from build123d import *

# Parameters (mm, degrees)
SKETCH1_R               = 3.25
BOSS_EXTRUDE1_DEPTH     = 1
SKETCH3_R               = 4.5
BOSS_EXTRUDE2_DEPTH     = 8
SKETCH4_W               = 43
SKETCH4_H               = 43
BOSS_EXTRUDE3_DEPTH     = 9
FILLET1_R               = 6
SKETCH5_R               = 12
BOSS_EXTRUDE4_DEPTH     = 14
CUT_EXTRUDE1_START      = 7
SKETCH6_R               = 12
SKETCH6_R_2             = 11
CUT_EXTRUDE1_DEPTH      = 1
BOSS_EXTRUDE5_DEPTH     = 3.5
FILLET2_R               = 4
SKETCH8_R               = 12
BOSS_EXTRUDE6_DEPTH     = 9
CHAMFER1_SIZE           = 1
BOSS_EXTRUDE7_START     = 10
SKETCH10_R              = 12
BOSS_EXTRUDE7_DEPTH     = 10
BOSS_EXTRUDE8_DEPTH     = 5
SKETCH12_R              = 12
BOSS_EXTRUDE9_DEPTH     = 48.5
CUT_EXTRUDE2_DEPTH      = 72.827221304
CUT_EXTRUDE2_DEPTH_BACK = 20
SKETCH13_W              = 26.789167307
SKETCH13_H              = 48.357994596
CHAMFER2_SIZE           = 1
CHAMFER4_SIZE           = 1
CHAMFER5_SIZE           = 1
SKETCH17_R              = 1.25
CUT_EXTRUDE4_DEPTH      = 88.387187875
CUT_EXTRUDE5_REACH      = 79.888
SKETCH18_R              = 3
SKETCH19_R              = 1.5
CUT_EXTRUDE6_DEPTH      = 53.140487552


with BuildPart() as part:
    # Sketch1 → Boss-Extrude1 (new body)
    with BuildSketch(Plane(origin=(0, 0, 0), x_dir=(1, 0, 0), z_dir=(0, 1, 0))):
        with BuildLine():
            Line((-17.5, -21.5), (17.5, -21.5))
            ThreePointArc((17.5, -21.5), (20.328427125, -20.328427125), (21.5, -17.5))
            Line((21.5, -17.5), (21.5, 17.5))
            ThreePointArc((21.5, 17.5), (20.328427125, 20.328427125), (17.5, 21.5))
            Line((17.5, 21.5), (-17.5, 21.5))
            ThreePointArc((-17.5, 21.5), (-20.328427125, 20.328427125), (-21.5, 17.5))
            Line((-21.5, 17.5), (-21.5, -17.5))
            ThreePointArc((-21.5, -17.5), (-20.328427125, -20.328427125), (-17.5, -21.5))
        make_face()
        with Locations(Location((-17.25, 17.25, 0), (0, 0, 270))):
            Circle(SKETCH1_R, mode=Mode.SUBTRACT)
        with Locations(Location((17.25, 17.25, 0), (0, 0, 270))):
            Circle(SKETCH1_R, mode=Mode.SUBTRACT)
        with Locations(Location((17.25, -17.25, 0), (0, 0, 270))):
            Circle(SKETCH1_R, mode=Mode.SUBTRACT)
        with Locations(Location((-17.25, -17.25, 0), (0, 0, 270))):
            Circle(SKETCH1_R, mode=Mode.SUBTRACT)
    extrude(amount=BOSS_EXTRUDE1_DEPTH)

    # Sketch3 → Boss-Extrude2 (add)
    with BuildSketch(Plane.XZ):
        with Locations(Location((-17.25, 17.25, 0), (0, 0, 70.811863546))):
            Circle(SKETCH3_R)
        with Locations(Location((17.25, 17.25, 0), (0, 0, 109.188136454))):
            Circle(SKETCH3_R)
        with Locations(Location((17.25, -17.25, 0), (0, 0, 19.188136454))):
            Circle(SKETCH3_R)
        with Locations(Location((-17.25, -17.25, 0), (0, 0, 160.811863546))):
            Circle(SKETCH3_R)
    extrude(amount=BOSS_EXTRUDE2_DEPTH)

    # Sketch4 → Boss-Extrude3 (add)
    with BuildSketch(Plane.XZ.offset(8)):
        Rectangle(SKETCH4_W, SKETCH4_H)
    extrude(amount=BOSS_EXTRUDE3_DEPTH)

    # Fillet1
    # the kernel refuses this fillet: 6 mm, written as the material it takes off along each edge
    with BuildSketch(Plane(origin=(-21.5, -8, 21.5), x_dir=(1, 0, 0), z_dir=(0, -1, 0)), Plane(origin=(-21.5, -8, -21.5), x_dir=(0, 0, 1), z_dir=(0, -1, 0)), Plane(origin=(21.5, -8, 21.5), x_dir=(0, 0, -1), z_dir=(0, -1, 0))) as fillet1_piece_1:
        with BuildLine():
            CenterArc((FILLET1_R, -FILLET1_R), FILLET1_R, 90, 90)
            Line((0, -FILLET1_R), (0, 0))
            Line((0, 0), (FILLET1_R, 0))
        make_face()
    extrude(amount=24, mode=Mode.SUBTRACT)
    with BuildSketch(Plane(origin=(21.5, -8, -21.5), x_dir=(0, 0, 1), z_dir=(0, -1, 0))) as fillet1_piece_2:
        with BuildLine():
            CenterArc((FILLET1_R, FILLET1_R), FILLET1_R, 180, 90)
            Line((0, FILLET1_R), (0, 0))
            Line((0, 0), (FILLET1_R, 0))
        make_face()
    extrude(amount=24, mode=Mode.SUBTRACT)

    # Sketch5 → Boss-Extrude4 (add)
    with BuildSketch(Plane.XZ.offset(17)):
        with Locations(Location((0, 0, 0), (0, 0, 270))):
            Circle(SKETCH5_R)
    extrude(amount=BOSS_EXTRUDE4_DEPTH)

    # Sketch6 → Cut-Extrude1 (cut)
    with BuildSketch(Plane.XZ.offset(17).offset(CUT_EXTRUDE1_START)):
        with Locations(Location((0, 0, 0), (0, 0, 270))):
            Circle(SKETCH6_R)
        with Locations(Location((0, 0, 0), (0, 0, 270))):
            Circle(SKETCH6_R_2, mode=Mode.SUBTRACT)
    extrude(amount=CUT_EXTRUDE1_DEPTH, mode=Mode.SUBTRACT)

    # Sketch7 → Boss-Extrude5 (add, symmetric)
    with BuildSketch(Plane(origin=(0, 0, 0), x_dir=(0, 0, -1), z_dir=(1, 0, 0))):
        Polygon((0, -25), (14.368756657, -25), (27.527515604, -41), (27.527515604, -66.788625846), (18.527515604, -66.788625846), (18.527515604, -41), (12, -31), (0, -31), align=None)
    extrude(amount=BOSS_EXTRUDE5_DEPTH, both=True)

    # Fillet2
    fillet2_edges = [part.edges().sort_by_distance(p)[0] for p in [
        (0, -31, -12),
    ]]
    fillet(fillet2_edges, radius=FILLET2_R)

    # Sketch8 → Boss-Extrude6 (add)
    with BuildSketch(Plane.XY.offset(-18.527515604)):
        with Locations((0, -55.310385562)):
            Circle(SKETCH8_R)
    extrude(amount=-BOSS_EXTRUDE6_DEPTH)

    # Chamfer1
    chamfer1_edges = [part.edges().sort_by_distance(p)[0] for p in [
        (0, -67.310385562, -18.527515604),
    ]]
    chamfer(chamfer1_edges, length=CHAMFER1_SIZE)

    # Sketch10 → Boss-Extrude7 (add)
    with BuildSketch(Plane.XY.offset(-18.527515604).offset(BOSS_EXTRUDE7_START)):
        with Locations(Location((0, -55.310385562, 0), (0, 0, 106.9577633))):
            Circle(SKETCH10_R)
    extrude(amount=-BOSS_EXTRUDE7_DEPTH)

    # Sketch11 → Boss-Extrude8 (add, symmetric)
    with BuildSketch(Plane(origin=(0, -55.310385562, 0), x_dir=(1, 0, 0), z_dir=(0, 1, 0))):
        Polygon((-13.638649199, -5.352201133), (-13.638649199, 8.527515604), (13.150518108, 8.527515604), (13.150518108, -5.352201133), (23.153950462, -5.352201133), (23.153950462, 14.212548323), (19.620962458, 18.527515604), (-23.642081553, 18.527515604), (-23.642081553, -5.352201133), align=None)
    extrude(amount=BOSS_EXTRUDE8_DEPTH, both=True)

    # Sketch12 → Boss-Extrude9 (add)
    with BuildSketch(Plane(origin=(23.153950462, 0, 0), x_dir=(0, 0, -1), z_dir=(1, 0, 0))):
        with Locations((-10.105239438, -55.310385562)):
            Circle(SKETCH12_R)
    extrude(amount=-BOSS_EXTRUDE9_DEPTH)

    # Sketch13 → Cut-Extrude2 (cut, two sides: drawn at the far end of the back side and taken through both)
    with BuildSketch(Plane.XZ.offset(60.310385562).offset(-CUT_EXTRUDE2_DEPTH_BACK)):
        with Locations((-0.244065546, 15.651481694)):
            Rectangle(SKETCH13_W, SKETCH13_H)
    extrude(amount=CUT_EXTRUDE2_DEPTH + CUT_EXTRUDE2_DEPTH_BACK, mode=Mode.SUBTRACT)

    # Chamfer2
    # the kernel refuses this chamfer: 2.030899419, 1 mm, written as the material it adds along each edge
    with BuildSketch(Plane(origin=(13.150518108, -50.310385562, -0.803472677), x_dir=(0, 0, -1), z_dir=(1, 0, 0)), Plane(origin=(-23.642081553, -50.310385562, -0.803472677), x_dir=(0, 0, -1), z_dir=(1, 0, 0))) as chamfer2_piece_1:
        with BuildLine():
            Line((CHAMFER2_SIZE, 0), (-1.730571797, 2.730571797))
            ThreePointArc((-1.730571797, 2.730571797), (-0.794397889, 1.45760387), (0, 0))
            Line((0, 0), (CHAMFER2_SIZE, 0))
        make_face()
    extrude(amount=10.003432354)

    # Chamfer4
    # the kernel refuses this chamfer: 2.030899419, 1 mm, written as the material it adds along each edge
    with BuildSketch(Plane(origin=(13.150518108, -60.310385562, -0.803472677), x_dir=(0, 0, -1), z_dir=(1, 0, 0))) as chamfer4_piece_1:
        with BuildLine():
            Line((CHAMFER4_SIZE, 0), (-1.730571797, -2.730571797))
            ThreePointArc((-1.730571797, -2.730571797), (-0.794397889, -1.45760387), (0, 0))
            Line((0, 0), (CHAMFER4_SIZE, 0))
        make_face()
    extrude(amount=10.003432354)

    # Chamfer5
    # the kernel refuses this chamfer: 2.030899419, 1 mm, written as the material it adds along each edge
    with BuildSketch(Plane(origin=(-23.642081553, -60.310385562, -0.803472677), x_dir=(0, 0, -1), z_dir=(1, 0, 0))) as chamfer5_piece_1:
        with BuildLine():
            Line((CHAMFER5_SIZE, 0), (-1.730571797, -2.730571797))
            ThreePointArc((-1.730571797, -2.730571797), (-0.794397889, -1.45760387), (0, 0))
            Line((0, 0), (CHAMFER5_SIZE, 0))
        make_face()
    extrude(amount=10.003432354)

    # Sketch17 → Cut-Extrude4 (cut, through all)
    with BuildSketch(Plane(origin=(0, 0, -27.527515604), x_dir=(-1, 0, 0), z_dir=(0, 0, -1))):
        with Locations(Location((0, -55.310385562, 0), (0, 0, 90))):
            Circle(SKETCH17_R)
    extrude(amount=-CUT_EXTRUDE4_DEPTH, mode=Mode.SUBTRACT)

    # Sketch18 → Cut-Extrude5 (cut, up to next)
    with BuildSketch(Plane(origin=(0, 1, 0), x_dir=(1, 0, 0), z_dir=(0, 1, 0)), mode=Mode.PRIVATE) as cut_extrude5_sk1:
        with Locations(Location((0, 0, 0), (0, 0, 270))):
            Circle(SKETCH18_R)
    cut_extrude5_tool1 = extrude(cut_extrude5_sk1.sketch, amount=-CUT_EXTRUDE5_REACH, mode=Mode.PRIVATE) & part.part
    add(cut_extrude5_tool1.solids().sort_by_distance((0, 1, 0))[0], mode=Mode.SUBTRACT)

    # Sketch19 → Cut-Extrude6 (cut, through all)
    with BuildSketch(Plane.XZ.offset(31)):
        with Locations(Location((0, 0, 0), (0, 0, 270))):
            Circle(SKETCH19_R)
    extrude(amount=-CUT_EXTRUDE6_DEPTH, mode=Mode.SUBTRACT)


solid = part.part
Verification items for the finished model (mm, model axes). A direction names the side the tool comes from. Give positions to 0.01 mm unless a question says otherwise; leave off trailing zeros. Loops run counter-clockwise (first coordinate to the right, second up) from the corner with the lowest first, then second, coordinate; pieces in that order, holes last. Notation, with made-up numbers: (59, 1.5) - (88, 1.5) arc R14 cw to (88, 5.5) - close; hole circle Ø8 at (46, 7). An arc over 180 degrees is marked (long way). Write each question's results on one line, items separated by ' | '.
1) Sectioned sample at B-B on z = -7. Record the boundary of the cut face in (x, y).
Solution:
outline: (-23.64, -60.31) - (-13.64, -60.31) - (-13.64, -50.31) - (-23.64, -50.31) - close; (-21.5, -17) - (-9.75, -17) - (-9.75, -24) - (-8.49, -24) - (-8.49, -25) - (-9.75, -25) - (-9.75, -31) - (9.75, -31) - (9.75, -25) - (8.49, -25) - (8.49, -24) - (9.75, -24) - (9.75, -17) - (21.5, -17) - (21.5, -8) - (-21.5, -8) - close; (-21.5, 0) - (21.5, 0) - (21.5, 1) - (-21.5, 1) - close; (13.15, -60.31) - (23.15, -60.31) - (23.15, -50.31) - (13.15, -50.31) - close
2) Depth check by flat-ended pin: P1, Ø5, axis at x = -18, z = -18.5, coming from the -Y side; P2, Ø0.8, axis at x = 8, y = 0.5, coming from the +Z side; P3, Ø1.5, axis at x = -4.5, y = -12.5, coming from the -Z side. Enter the tip coordinate at first touch or a pass-through.
Solution:
P1: y = -60.31 | P2: z = 21.5 | P3: z = -21.5
3) Sectioned sample at A-A on y = -10.5. Record the boundary of the cut face in (x, z).
Solution:
outline: (-21.5, -15.5) arc R6 ccw to (-15.5, -21.5) - (15.5, -21.5) arc R6 ccw to (21.5, -15.5) - (21.5, 15.5) arc R6 ccw to (15.5, 21.5) - (-15.5, 21.5) arc R6 ccw to (-21.5, 15.5) - close; hole circle Ø3 at (0, 0)
4) Mould release check, pull along Y, two halves, no side actions. Record for faces 1 (the flat face through (0, -42, -18.528)), 2 (the flat face through (18.082, -61.657, -0.457)), 3 (the cylindrical face through (20.359, 0.493, -20.297)), 4 (the cylindrical face through (-20.78, -3.94, -20.04)): pulls with the +Y half, pulls with the -Y half, needs draft (parallel to the pull), parting line crosses it, or undercut.
Solution:
face 1: undercut | face 2: pulls with the -Y half | face 3: needs draft | face 4: undercut
5) Sectioned sample at C-C on x = -19. Count the separate pieces of the cut face and the enclosed holes in it, plus the area to 3 significant figures.
Solution:
separate pieces: 2 | enclosed holes: 1 | area: 1,160 mm2
6) Material ranges on L1, parallel to Y at x = 12.5, z = -11.5; L2, parallel to X at y = 0.7, z = 17.25; L3, parallel to Y at x = -10, z = -5, recorded low to high. Write a range as from..to.
Solution:
L1: -60.31..-50.31, -17..-8, 0..1 | L2: -21.5..-20.5, -14..14, 20.5..21.5 | L3: -31..-25, -24..-8, 0..1
7) Tool access check on faces 5 (the flat face through (-20, -8, -20)), 6 (the flat face through (0.05, -36.96, -15.89)), 7 (the cylindrical face through (20.297, 0.493, 20.359)). Record the directions out of +Z, -Z, +X, -X, +Y, -Y that give a thin tool (end or side, any length) a straight path to the whole face; none if there is none.
Solution:
face 5: -Z, -X | face 6: +Z, +X, -X | face 7: +Z, +X, +Y
